from build123d import *

# Parameters (mm, degrees)
SKETCH1_R           = 1.5
BOSS_EXTRUDE1_DEPTH = 5
BOSS_EXTRUDE2_DEPTH = 20
CUT_EXTRUDE1_REACH  = 84.141
SKETCH3_R           = 1.5


with BuildPart() as part:
    # Sketch1 → Boss-Extrude1 (new body)
    with BuildSketch(Plane(origin=(0, 0, 0), x_dir=(1, 0, 0), z_dir=(0, 1, 0))):
        Polygon((-14.2078125, 0), (14.2078125, 0), (19.2078125, 5), (19.2078125, 19.525), (24.2078125, 24.525), (45, 24.525), (50, 29.525), (50, 72.025), (40, 72.025), (40, 69.953932188), (35, 64.953932188), (-35, 64.953932188), (-40, 69.953932188), (-40, 72.025), (-50, 72.025), (-50, 29.525), (-45, 24.525), (-24.2078125, 24.525), (-19.2078125, 19.525), (-19.2078125, 5), align=None)
        with Locations(Location((45, 34.525, 0), (0, 0, 270))):
            Circle(SKETCH1_R, mode=Mode.SUBTRACT)
        with Locations(Location((45, 47.025, 0), (0, 0, 270))):
            Circle(SKETCH1_R, mode=Mode.SUBTRACT)
        with Locations(Location((45, 62.025, 0), (0, 0, 270))):
            Circle(SKETCH1_R, mode=Mode.SUBTRACT)
        with Locations(Location((-45, 62.025, 0), (0, 0, 90))):
            Circle(SKETCH1_R, mode=Mode.SUBTRACT)
        with Locations(Location((-45, 47.025, 0), (0, 0, 90))):
            Circle(SKETCH1_R, mode=Mode.SUBTRACT)
        with Locations(Location((-45, 34.525, 0), (0, 0, 90))):
            Circle(SKETCH1_R, mode=Mode.SUBTRACT)
        Polygon((-9.525, 10), (9.525, 10), (9.525, 15.953125), (11.7078125, 15.953125), (11.7078125, 19.525), (-11.7078125, 19.525), (-11.7078125, 15.953125), (-9.525, 15.953125), align=None, mode=Mode.SUBTRACT)
        Polygon((2.5, 54.953932188), (2.5, 29.525), (32.928932188, 59.953932188), (7.5, 59.953932188), align=None, mode=Mode.SUBTRACT)
        Polygon((40, 59.953932188), (9.571067812, 29.525), (35, 29.525), (40, 34.525), align=None, mode=Mode.SUBTRACT)
        Polygon((-40, 34.525), (-40, 59.953932188), (-9.571067812, 29.525), (-35, 29.525), align=None, mode=Mode.SUBTRACT)
        Polygon((-2.5, 29.525), (-32.928932188, 59.953932188), (-7.5, 59.953932188), (-2.5, 54.953932188), align=None, mode=Mode.SUBTRACT)
    extrude(amount=BOSS_EXTRUDE1_DEPTH)

    # Sketch2 → Boss-Extrude2 (add)
    with BuildSketch(Plane(origin=(0, 0, 0), x_dir=(1, 0, 0), z_dir=(0, 1, 0))):
        Polygon((19.2078125, 19.525), (19.2078125, 5), (14.2078125, 0), (-14.2078125, 0), (-19.2078125, 5), (-19.2078125, 19.525), (-16.7078125, 22.025), (-9.525, 22.025), (-9.525, 19.525), (-11.7078125, 19.525), (-11.7078125, 15.953125), (-9.525, 15.953125), (-9.525, 10), (9.525, 10), (9.525, 15.953125), (11.7078125, 15.953125), (11.7078125, 19.525), (9.525, 19.525), (9.525, 22.025), (16.7078125, 22.025), align=None)
    extrude(amount=-BOSS_EXTRUDE2_DEPTH)

    # Sketch3 → Cut-Extrude1 (cut, up to next)
    with BuildSketch(Plane(origin=(0, 0, -10), x_dir=(-1, 0, 0), z_dir=(0, 0, -1)), mode=Mode.PRIVATE) as cut_extrude1_sk1:
        with Locations((0, -15)):
            Circle(SKETCH3_R)
    cut_extrude1_tool1 = extrude(cut_extrude1_sk1.sketch, amount=-CUT_EXTRUDE1_REACH, mode=Mode.PRIVATE) & part.part
    # Sketch3 → Cut-Extrude1 (cut, up to next)
    with BuildSketch(Plane(origin=(0, 0, -10), x_dir=(-1, 0, 0), z_dir=(0, 0, -1)), mode=Mode.PRIVATE) as cut_extrude1_sk2:
        with Locations((0, -5)):
            Circle(SKETCH3_R)
    cut_extrude1_tool2 = extrude(cut_extrude1_sk2.sketch, amount=-CUT_EXTRUDE1_REACH, mode=Mode.PRIVATE) & part.part
    add(cut_extrude1_tool1.solids().sort_by_distance((0, -15, -10))[0], mode=Mode.SUBTRACT)
    add(cut_extrude1_tool2.solids().sort_by_distance((0, -5, -10))[0], mode=Mode.SUBTRACT)


solid = part.part
The listing builds one solid part. Answer for the finished solid, in the listing's coordinates (mm). A direction names the side the tool comes from. Give positions to 0.01 mm unless a question says otherwise; leave off trailing zeros. Loops run counter-clockwise (first coordinate to the right, second up) from the corner with the lowest first, then second, coordinate; pieces in that order, holes last. Notation, with made-up numbers: (-37.5, 40) - (-28.5, 40) arc R20 cw to (-28.5, 67) - close; hole circle Ø5 at (5.25, 35.5). An arc over 180 degrees is marked (long way). Write each question's results on one line, items separated by ' | '.
1. Find section D-D, the plane x = 28. Write down the section's boundary in (y, z) (3 decimals), then the cut area to 3 significant figures.
Resolved:
outline: (0, -64.954) - (5, -64.954) - (5, -59.954) - (0, -59.954) - close; (0, -55.025) - (5, -55.025) - (5, -47.954) - (0, -47.954) - close; (0, -29.525) - (5, -29.525) - (5, -24.525) - (0, -24.525) - close | area: 85.4 mm^2
2. Consider probe 1 along Z at (x, y) = (-45, 1.55) (3 decimals); probe 2 along Y at (x, z) = (0, -4); probe 3 along X at (y, z) = (-14.5, -16.5). Determine where each line is inside the solid, lowest interval first. Write a range as from..to.
Resolved:
probe 1: z = -72.025..-63.525, -60.525..-48.525, -45.525..-36.025, -33.025..-24.525 | probe 2: y = -20..-16.5, -13.5..-6.5, -3.5..5 | probe 3: x = -19.21..-11.71, 11.71..19.21
3. Find section A-A, the plane y = -15. Write down the section's boundary in (x, z) (3 decimals).
Resolved:
outline: (-19.208, -19.525) - (-16.708, -22.025) - (-9.525, -22.025) - (-9.525, -19.525) - (-11.708, -19.525) - (-11.708, -15.953) - (-9.525, -15.953) - (-9.525, -10) - (-1.5, -10) - (-1.5, 0) - (-14.208, 0) - (-19.208, -5) - close; (1.5, -10) - (9.525, -10) - (9.525, -15.953) - (11.708, -15.953) - (11.708, -19.525) - (9.525, -19.525) - (9.525, -22.025) - (16.708, -22.025) - (19.208, -19.525) - (19.208, -5) - (14.208, 0) - (1.5, 0) - close
4. For a pull along X with two mould halves and no side action, classify faces 6 (the face through (-13, -10, -22.025)), 7 (the face through (-16.673, -7.325, -2.465)), 8 (the face through (-44.087, 2.465, -60.835)) as +X half, -X half, draft (parallel to the pull), parting line (faces both ways), or undercut.
Resolved:
face 6: draft | face 7: -X half | face 8: undercut
5. Find section C-C, the plane z = -52. Write down the section's boundary in (x, y) (3 decimals), then the cut area to 3 significant figures.
Resolved:
outline: (-50, 0) - (-40, 0) - (-40, 5) - (-50, 5) - close; (-32.046, 0) - (-24.975, 0) - (-24.975, 5) - (-32.046, 5) - close; (-2.5, 0) - (2.5, 0) - (2.5, 5) - (-2.5, 5) - close; (24.975, 0) - (32.046, 0) - (32.046, 5) - (24.975, 5) - close; (40, 0) - (50, 0) - (50, 5) - (40, 5) - close | area: 196 mm^2
6. Which of the six approach directions +Z, -Z, +X, -X, +Y, -Y give full straight-line access (tool end or side, diameter ignored) to faces 1 (the face through (-22, 2, -29.525)), 2 (the face through (13, -10, -22.025)), 3 (the face through (9.525, -10, -21)), 4 (the face through (34, 2, -24.525)), 5 (the face through (0.325, -16.464, -5.07))?
Resolved:
face 1: +Y, -Y | face 2: -Z, +X, -X, -Y | face 3: -Z, -Y | face 4: +Z, +X, +Y, -Y | face 5: +Z, -Z
7. Flat-ended cylindrical pins translate along their axes: P1, Ø5, axis at y = -6, z = -14, coming from the +X side; P2, Ø1.7, axis at x = 11, y = -8, coming from the -Z side (3 decimals); P3, Ø1, axis at x = -40, z = -42, coming from the -Y side; P4, Ø2, axis at x = 4, z = -46, coming from the +Y side. Find the tip coordinate at first contact, or state that the pin passes through.
Resolved:
P1: stops at x = 19.21 | P2: stops at z = -22.025 | P3: stops at y = 0 | P4: passes through
8. Find section B-B, the plane x = 0. Write down the section's boundary in (y, z) (3 decimals), then the cut area to 3 significant figures.
Resolved:
outline: (-20, -10) - (-16.5, -10) - (-16.5, 0) - (-20, 0) - close; (-13.5, -10) - (-6.5, -10) - (-6.5, 0) - (-13.5, 0) - close; (-3.5, -10) - (5, -10) - (5, 0) - (-3.5, 0) - close; (0, -64.954) - (5, -64.954) - (5, -19.525) - (0, -19.525) - close | area: 417 mm^2
